Read the model definition and answer for the solid it produces. Units are mm, in the model's axes. Face numbers are marked on the shaded views. A direction names the side the tool comes from. Coordinates: 2 decimals unless noted, no trailing zeros. Order: outer loops, then holes, each group sorted by start corner. A loop starts at its lowest first (then second) coordinate and runs counter-clockwise, first axis right, second up. Notation, with made-up numbers: M 69.5,71.5 L 103.5,71.5 A18 cw 103.5,106.5 Z; hole C 55.25,70 d6. An arc over 180 degrees is marked long. One line per question, with ' | ' between items. Start each with the question number.
1) Find section B-B, the plane z = 2. Write down the section's boundary in (x, y), plus the area to 3 significant figures.
2) A tool of negligible diameter and unlimited length cuts with its end or side. For the marked faces 4 and 5, from which of +Z, -Z, +X, -X, +Y, -Y can it reach the whole face along a straight path? Write none if from no direction.
3) Find section D-D, the plane z = 14.5. Write down the section's boundary in (x, y).
4) The mould has two halves that part along X. Classify the marked faces 1, 2 and 3: +X half, -X half, draft (parallel to the pull), parting line (faces both ways), or undercut.
5) Consider probe 1 along X at (y, z) = (12, 2); probe 2 along Z at (x, y) = (16, 22); probe 3 along X at (y, z) = (22, 10.5). Determine where each line is inside the solid, lowest interval first.
6) Given P1, Ø10, axis at y = 22, z = 6.5, coming from the -X side; P2, Ø4.5, axis at x = 4.61, z = 15.5, coming from the +Y side; P3, Ø2, axis at x = 5, y = 1, coming from the +Z side; P4, Ø10, axis at x = -9, y = 8, coming from the +Z side, each flat-ended and moving along its own axis, determine where each tip first touches the part or whether it passes through.
7) Find section C-C, the plane y = 13. Write down the section's boundary in (x, z), plus the area to 3 significant figures.
8) Find section A-A, the plane x = 1. Write down the section's boundary in (y, z), plus the area to 3 significant figures.
from build123d import *

# Parameters (mm, degrees)
SKETCH1_W             = 20
SKETCH1_H             = 8
SKETCH1_R             = 2
BOSS_EXTRUDE1_DEPTH   = 2
BOSS_EXTRUDE1_2_DEPTH = 2
SKETCH6_W             = 56
SKETCH6_H             = 2
BOSS_EXTRUDE5_DEPTH   = 6
SKETCH10_W            = 56
SKETCH10_H            = 2
BOSS_EXTRUDE7_DEPTH   = 4
SKETCH11_W            = 56.175194469
SKETCH11_H            = 14.528307745
BOSS_EXTRUDE8_DEPTH   = 2
SKETCH12_R            = 2.5
CUT_EXTRUDE3_DEPTH    = 2
SKETCH13_W            = 20
SKETCH13_H            = 50
BOSS_EXTRUDE9_DEPTH   = 2


with BuildPart() as part:
    # Sketch1 → Boss-Extrude1 (new body)
    with BuildSketch(Plane(origin=(0, 0, 0), x_dir=(1, 0, 0), z_dir=(0, 1, 0))):
        with Locations((-0.385906166, -15.501316712)):
            Rectangle(SKETCH1_W, SKETCH1_H)
        with Locations(Location((4.614093834, -15.501316712, 0), (0, 0, 270))):
            Circle(SKETCH1_R, mode=Mode.SUBTRACT)
        with Locations(Location((-5.385906166, -15.501316712, 0), (0, 0, 270))):
            Circle(SKETCH1_R, mode=Mode.SUBTRACT)
    extrude(amount=BOSS_EXTRUDE1_DEPTH)



with BuildPart() as body_2:
    # Sketch1 → Boss-Extrude1 2 (new body)
    with BuildSketch(Plane(origin=(0, 0, 0), x_dir=(1, 0, 0), z_dir=(0, 1, 0))):
        with Locations((-0.385906166, 32.498683288)):
            Rectangle(SKETCH1_W, SKETCH1_H)
        with Locations(Location((4.614093834, 32.498683288, 0), (0, 0, 270))):
            Circle(SKETCH1_R, mode=Mode.SUBTRACT)
        with Locations(Location((-5.385906166, 32.498683288, 0), (0, 0, 270))):
            Circle(SKETCH1_R, mode=Mode.SUBTRACT)
    extrude(amount=BOSS_EXTRUDE1_2_DEPTH)


with BuildPart() as part_1:
    add(part.part)

    add(body_2.part)  # Boss-Extrude5 merges body 2
    # Sketch6 → Boss-Extrude5 (add)
    with BuildSketch(Plane(origin=(9.614093834, 0, 0), x_dir=(0, 0, -1), z_dir=(1, 0, 0))):
        with Locations((8.498683288, 1)):
            Rectangle(SKETCH6_W, SKETCH6_H)
    extrude(amount=BOSS_EXTRUDE5_DEPTH)

    # Sketch10 → Boss-Extrude7 (add)
    with BuildSketch(Plane.ZY.offset(10.385906166)):
        with Locations((-8.498683288, 1)):
            Rectangle(SKETCH10_W, SKETCH10_H)
    extrude(amount=BOSS_EXTRUDE7_DEPTH)

    # Sketch11 → Boss-Extrude8 (add)
    with BuildSketch(Plane.ZY.offset(14.385906166)):
        with Locations((-8.411086054, 7.264153873)):
            Rectangle(SKETCH11_W, SKETCH11_H)
    extrude(amount=BOSS_EXTRUDE8_DEPTH)

    # Sketch12 → Cut-Extrude3 (cut)
    with BuildSketch(Plane.ZY.offset(16.385906166)):
        with Locations((-8.411086053, 8.528307745)):
            Circle(SKETCH12_R)
    extrude(amount=-CUT_EXTRUDE3_DEPTH, mode=Mode.SUBTRACT)

    # Sketch13 → Boss-Extrude9 (add)
    with BuildSketch(Plane(origin=(15.614093834, 0, 0), x_dir=(0, 0, -1), z_dir=(1, 0, 0))):
        with Locations((-1.501316712, 17)):
            Rectangle(SKETCH13_W, SKETCH13_H)
    extrude(amount=BOSS_EXTRUDE9_DEPTH)


solid = part_1.part
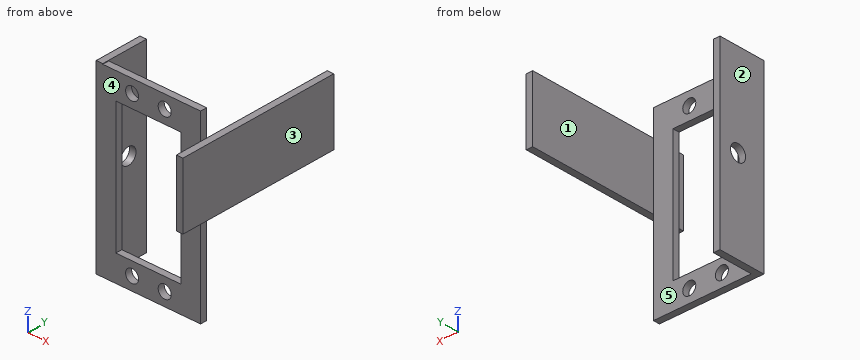
Report:
1) outline: M -16.39,0 L -10.39,0 L -10.39,2 L -14.39,2 L -14.39,14.53 L -16.39,14.53 Z; M 9.61,0 L 15.61,0 L 15.61,-8 L 17.61,-8 L 17.61,42 L 15.61,42 L 15.61,2 L 9.61,2 Z | area: 149 mm^2
2) face 4: +Z, -Z, -X, -Y | face 5: +Z, -Z, +Y
3) outline: M -16.39,0 L -7.12,0 L -7.12,2 L -14.39,2 L -14.39,14.53 L -16.39,14.53 Z; M -3.65,0 L 2.88,0 L 2.88,2 L -3.65,2 Z; M 6.35,0 L 15.61,0 L 15.61,2 L 6.35,2 Z
4) face 1: undercut | face 2: -X half | face 3: +X half
5) probe 1: x = -16.39 to -14.39, 15.61 to 17.61 | probe 2: z = -8.5 to 11.5 | probe 3: x = 15.61 to 17.61
6) P1: stops at x = 15.61 | P2: stops at y = 2 | P3: stops at z = 19.5 | P4: passes through
7) outline: M -16.39,-36.5 L -14.39,-36.5 L -14.39,19.68 L -16.39,19.68 Z; M 15.61,-8.5 L 17.61,-8.5 L 17.61,11.5 L 15.61,11.5 Z | area: 152 mm^2
8) outline: M 0,-36.5 L 2,-36.5 L 2,-28.5 L 0,-28.5 Z; M 0,11.5 L 2,11.5 L 2,19.5 L 0,19.5 Z | area: 32.0 mm^2
